Source: CAD feature listing. Evaluate the final solid. Frame: model axes, mm. Face numbers are marked on the shaded views. Round coordinates to 2 decimals unless told otherwise and drop trailing zeros. Loops run counter-clockwise (first coordinate to the right, second up) from the corner with the lowest first, then second, coordinate; pieces in that order, holes last. Notation, with made-up numbers: M -20,-11.75 L -15,-11.75 A14 cw -15,4.25 Z; hole C 12,67.5 d8. An arc over 180 degrees is marked long. One line per item, written item: value.
from build123d import *

# Parameters (mm, degrees)
SKETCH1_W           = 45
SKETCH1_H           = 25
BOSS_EXTRUDE1_DEPTH = 12
SKETCH2_R           = 2.5
CUT_EXTRUDE1_DEPTH  = 12
SKETCH3_R           = 2.5
CUT_EXTRUDE2_DEPTH  = 72
SKETCH4_R           = 2.5
CUT_EXTRUDE3_DEPTH  = 72
SKETCH5_R           = 6
CUT_EXTRUDE4_DEPTH  = 72
SKETCH6_R           = 2.5
CUT_EXTRUDE5_DEPTH  = 72
SKETCH7_R           = 2.5
BOSS_EXTRUDE2_DEPTH = 12


with BuildPart() as part:
    # Sketch1 → Boss-Extrude1 (new body)
    with BuildSketch(Plane(origin=(0, 0, 0), x_dir=(1, 0, 0), z_dir=(0, 1, 0))):
        Rectangle(SKETCH1_W, SKETCH1_H)
    extrude(amount=BOSS_EXTRUDE1_DEPTH)

    # Sketch2 → Cut-Extrude1 (cut)
    with BuildSketch(Plane(origin=(0, 12, 0), x_dir=(1, 0, 0), z_dir=(0, 1, 0))):
        with Locations((-18, -7.5)):
            Circle(SKETCH2_R)
        with Locations((-18, 7.5)):
            Circle(SKETCH2_R)
        with Locations((18, -7.5)):
            Circle(SKETCH2_R)
        with Locations((18, 7.5)):
            Circle(SKETCH2_R)
    extrude(amount=-CUT_EXTRUDE1_DEPTH, mode=Mode.SUBTRACT)

    # Sketch3 → Cut-Extrude2 (cut)
    with BuildSketch(Plane(origin=(0, 0, -12.5), x_dir=(-1, 0, 0), z_dir=(0, 0, -1))):
        with Locations((0, 6)):
            Circle(SKETCH3_R)
    extrude(amount=-CUT_EXTRUDE2_DEPTH, mode=Mode.SUBTRACT)

    # Sketch4 → Cut-Extrude3 (cut)
    with BuildSketch(Plane(origin=(0, 0, -12.5), x_dir=(-1, 0, 0), z_dir=(0, 0, -1))):
        with Locations((10, 6)):
            Circle(SKETCH4_R)
        with Locations((-10, 6)):
            Circle(SKETCH4_R)
    extrude(amount=-CUT_EXTRUDE3_DEPTH, mode=Mode.SUBTRACT)

    # Sketch5 → Cut-Extrude4 (cut)
    with BuildSketch(Plane(origin=(0, 12, 0), x_dir=(1, 0, 0), z_dir=(0, 1, 0))):
        Circle(SKETCH5_R)
    extrude(amount=-CUT_EXTRUDE4_DEPTH, mode=Mode.SUBTRACT)

    # Sketch6 → Cut-Extrude5 (cut)
    with BuildSketch(Plane(origin=(0, 12, 0), x_dir=(1, 0, 0), z_dir=(0, 1, 0))):
        with Locations((-18, 0)):
            Circle(SKETCH6_R)
        with Locations((18, 0)):
            Circle(SKETCH6_R)
    extrude(amount=-CUT_EXTRUDE5_DEPTH, mode=Mode.SUBTRACT)

    # Sketch7 → Boss-Extrude2 (add)
    with BuildSketch(Plane(origin=(0, 12, 0), x_dir=(1, 0, 0), z_dir=(0, 1, 0))):
        with Locations((18, -7.5)):
            Circle(SKETCH7_R)
        with Locations((18, 7.5)):
            Circle(SKETCH7_R)
        with Locations((-18, -7.5)):
            Circle(SKETCH7_R)
        with Locations((-18, 7.5)):
            Circle(SKETCH7_R)
    extrude(amount=-BOSS_EXTRUDE2_DEPTH)


solid = part.part
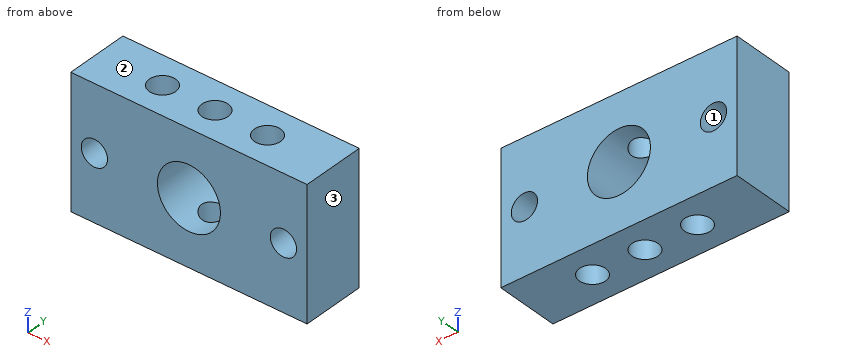
1. Section query B-B (z = 10). Return the cut outline in (x, y), and give its area (3 significant figures).
Report:
outline: M -22.5,0 L 22.5,0 L 22.5,12 L -22.5,12 Z; hole C -10,6 d5; hole C 0,6 d5; hole C 10,6 d5
area: 481 mm2
2. Section query C-C (x = 0). Return the cut outline in (y, z), and give its area (3 significant figures).
Report:
outline: M 0,-12.5 L 3.5,-12.5 L 3.5,-6 L 0,-6 Z; M 0,6 L 3.5,6 L 3.5,12.5 L 0,12.5 Z; M 8.5,-12.5 L 12,-12.5 L 12,-6 L 8.5,-6 Z; M 8.5,6 L 12,6 L 12,12.5 L 8.5,12.5 Z
area: 91.0 mm2
3. Ray query, line 1 (X direction, y = 9.5, z = 0); line 2 (X direction, y = 11.5, z = 2); line 3 (Z direction, x = -2.5, y = 1.5). Return the intervals inside material, ascending. Write a range as [from, to].
Report:
line 1: x = [-22.5, -20.5], [-15.5, -6], [6, 15.5], [20.5, 22.5]
line 2: x = [-22.5, -19.5], [-16.5, -5.66], [5.66, 16.5], [19.5, 22.5]
line 3: z = [-12.5, -5.45], [5.45, 12.5]
4. Pull-direction query (Z, two-part tool) for the marked faces 1, 2 and 3; classes: released by +Z, released by -Z, zero draft, split by the parting line, or undercut.
Report:
face 1: undercut
face 2: released by +Z
face 3: zero draft
5. Section query D-D (z = 0). Return the cut outline in (x, y).
Report:
outline: M -22.5,0 L -20.5,0 L -20.5,12 L -22.5,12 Z; M -15.5,0 L -6,0 L -6,12 L -15.5,12 Z; M 6,0 L 15.5,0 L 15.5,12 L 6,12 Z; M 20.5,0 L 22.5,0 L 22.5,12 L 20.5,12 Z; hole C -10,6 d5; hole C 10,6 d5
6. Section query A-A (y = 6). Return the cut outline in (x, z).
Report:
outline: M -22.5,-12.5 L -12.5,-12.5 L -12.5,12.5 L -22.5,12.5 Z; M -7.5,-12.5 L -2.5,-12.5 L -2.5,-5.45 A6 cw -2.5,5.45 L -2.5,12.5 L -7.5,12.5 Z; M 2.5,-12.5 L 7.5,-12.5 L 7.5,12.5 L 2.5,12.5 L 2.5,5.45 A6 cw 2.5,-5.45 Z; M 12.5,-12.5 L 22.5,-12.5 L 22.5,12.5 L 12.5,12.5 Z; hole C -18,0 d5; hole C 18,0 d5
